For this review, take the finished solid that the model builds, in its own axes (mm). Give positions to 0.01 mm unless a question says otherwise; leave off trailing zeros. Order: outer loops, then holes, each group sorted by start corner. A loop starts at its lowest first (then second) coordinate and runs counter-clockwise, first axis right, second up. Notation, with made-up numbers: M 19,29 L 42,29 A9 cw 42,39 Z; hole C -22.5,7.5 d9. An arc over 180 degrees is marked long. Use CSV: the item, a comma, the result in double quotes. Start each with the question number.
(1) Consider section B-B (z = 0). Write out the cut boundary in (x, y).
(2) Wall thickness on L1, parallel to X at y = 3.05, z = 0; L2, parallel to X at y = 1.65, z = -13.5: over which ranges is each line inside the solid? List them lowest first. Write a range as from..to.
(3) Consider section C-C (y = 1.85). Give the number of separate pieces and of enclosed holes in the cut face, and give its area (3 significant figures).
(4) Draft analysis for pull direction Z (two halves, no side actions). For faces 1 (the face through (23.846, 2.958, -7.509)), 2 (the face through (14.77, 2.96, -13.25)), 3 (the face through (19.9, 3, 1.2)), 4 (the face through (5, 6, 5)), state which applies: pulls with the +Z half, pulls with the -Z half, needs draft (parallel to the pull), parting line crosses it, or undercut.
(5) Consider section D-D (x = 20.5). Write out the cut boundary in (y, z).
(6) Clearance check with flat-ended pins moving along their axes: P1, Ø6.5, axis at x = 15.2, z = 15.2, coming from the -Y side; P2, Ø2, axis at x = -3.5, y = 3.5, coming from the -Z side; P3, Ø1.5, axis at x = -14.5, y = 4.5, coming from the +Z side. State where each tip first meets the part, or that it passes through.
(7) Consider section A-A (x = 0). Write out the cut boundary in (y, z).
```python
from build123d import *

# Parameters (mm, degrees)
SKETCH_1_R      = 25
SKETCH_1_R_2    = 2
SKETCH_1_R_3    = 6.260668566
EXTRUDE_1_DEPTH = 6


with BuildPart() as part:
    # 草图1 → 凸台-拉伸1 (new body)
    with BuildSketch(Plane(origin=(0, 0, 0), x_dir=(1, 0, 0), z_dir=(0, 1, 0))):
        Circle(SKETCH_1_R)
        with Locations((0, 21.5)):
            Circle(SKETCH_1_R_2, mode=Mode.SUBTRACT)
        with Locations((15.202795796, 15.202795796)):
            Circle(SKETCH_1_R_2, mode=Mode.SUBTRACT)
        with Locations((21.5, 0)):
            Circle(SKETCH_1_R_2, mode=Mode.SUBTRACT)
        with Locations((15.202795796, -15.202795796)):
            Circle(SKETCH_1_R_2, mode=Mode.SUBTRACT)
        with Locations((0, -21.5)):
            Circle(SKETCH_1_R_2, mode=Mode.SUBTRACT)
        with Locations((-15.202795796, -15.202795796)):
            Circle(SKETCH_1_R_2, mode=Mode.SUBTRACT)
        with Locations((-21.5, 0)):
            Circle(SKETCH_1_R_2, mode=Mode.SUBTRACT)
        with Locations((-15.202795796, 15.202795796)):
            Circle(SKETCH_1_R_2, mode=Mode.SUBTRACT)
        Circle(SKETCH_1_R_3, mode=Mode.SUBTRACT)
    extrude(amount=EXTRUDE_1_DEPTH)


solid = part.part
```
Check result:
1,outline,"M -25,0 L -23.5,0 L -23.5,6 L -25,6 Z; M -19.5,0 L -6.26,0 L -6.26,6 L -19.5,6 Z; M 6.26,0 L 19.5,0 L 19.5,6 L 6.26,6 Z; M 23.5,0 L 25,0 L 25,6 L 23.5,6 Z"
2,L1,"x = -25..-23.5, -19.5..-6.26, 6.26..19.5, 23.5..25"
2,L2,"x = -21.04..-16.25, -14.15..14.15, 16.25..21.04"
3,separate pieces,"1"
3,enclosed holes,"9"
3,area,"1,740 mm^2"
4,face 1,"parting line crosses it"
4,face 2,"undercut"
4,face 3,"undercut"
4,face 4,"needs draft"
5,outline,"M 0,-14.31 L 6,-14.31 L 6,-1.73 L 0,-1.73 Z; M 0,1.73 L 6,1.73 L 6,14.31 L 0,14.31 Z"
6,P1,"stops at y = 0"
6,P2,"stops at z = -24.87"
6,P3,"stops at z = 20.88"
7,outline,"M 0,-25 L 6,-25 L 6,-23.5 L 0,-23.5 Z; M 0,-19.5 L 6,-19.5 L 6,-6.26 L 0,-6.26 Z; M 0,6.26 L 6,6.26 L 6,19.5 L 0,19.5 Z; M 0,23.5 L 6,23.5 L 6,25 L 0,25 Z"
